Part model, mm, in its own coordinate system. A direction names the side the tool comes from. Give positions to 0.01 mm unless a question says otherwise; leave off trailing zeros. Order: outer loops, then holes, each group sorted by start corner. A loop starts at its lowest first (then second) coordinate and runs counter-clockwise, first axis right, second up. Notation, with made-up numbers: (73.5, -21.5) - (88.5, -21.5) arc R24 cw to (88.5, 10.5) - close; hole circle Ø2 at (31.5, 32). An arc over 180 degrees is marked (long way). Use one line per item in the form item = value. Start each with the question number.
1. Pull direction Z, two halves, no side cores. Call faces 4 (the face through (0, 2, 27.5)), 5 (the face through (10.927, 2, -20)), 6 (the face through (7.25, 2, -11)): +Z half, -Z half, draft (parallel to the pull), parting line (faces both ways), or undercut.
2. Drill centre lines: line 1 (Z direction, x = -7.5, y = 3.6); line 2 (X direction, y = 0.4, z = 5.5). Where is each one in solid material? Low to high.
3. Band-saw the part on A-A, the plane x = -8.25. List the corners of the cut face in (y, z).
4. Band-saw the part on C-C, the plane z = 13. List the corners of the cut face in (x, y).
5. Tool access for faces 1 (the face through (9, 2, -15.5)), 2 (the face through (-9, 2, 14.5)), 3 (the face through (-9, 2, 24.5)): list every direction of +Z, -Z, +X, -X, +Y, -Y with a clear straight run to the whole face (end or side of a thin tool).
6. Pin check, flat tips, straight feed: P1, Ø4, axis at x = -1.5, z = 3, coming from the -Y side; P2, Ø1.9, axis at x = -9.5, y = 1.5, coming from the +Z side; P3, Ø0.9, axis at y = 1, z = 26, coming from the +X side; P4, Ø1.2, axis at y = 2.5, z = -8.5, coming from the -X side. Stop position of each tip, or through.
7. Band-saw the part on B-B, the plane y = 2. List the corners of the cut face in (x, z), plus the area to 3 significant figures.
Autodesk Inventor part; units mm, degrees
ref_plane "YZ Plane" through (0, 0, 0) normal (1, 0, 0) x (0, 1, 0)
ref_plane "XZ Plane" through (0, 0, 0) normal (0, 1, 0) x (-1, 0, 0)
ref_plane "XY Plane" through (0, 0, 0) normal (0, 0, 1) x (1, 0, 0)
sketch "Sketch1" plane through (0, 0, 0) normal (0, 1, 0) x (-1, 0, 0)
  line L0 (-7.25, 27.5) -> (7.25, 27.5)
  line L1 (7.25, 27.5) -> (7.25, -27.5)
  line L2 (7.25, -27.5) -> (-7.25, -27.5)
  line L3 (-7.25, -27.5) -> (-7.25, 27.5)
  line L4 (-7.25, 27.5) -> (7.25, -27.5) construction
  line L5 (7.25, 27.5) -> (-7.25, -27.5) construction
  point P0 (0, 0)
  dimension "d0" = 14.5
  dimension "d1" = 55
extrude "Extrusion1" add sketch "Sketch1" along normal blind 4
sketch "Sketch2" plane through (0, 4, 0) normal (0, 1, 0) x (1, 0, 0)
  line L0 (0, -21.4425) -> (0, 24.9563)
  line L1 (6.9273, -24.5) -> (10.9273, -24.5)
  line L2 (10.9273, -24.5) -> (10.9273, -14.5)
  line L3 (10.9273, -14.5) -> (6.9273, -14.5)
  line L4 (6.9273, -14.5) -> (6.9273, -24.5)
  line L5 (7.25, -27.5) -> (-7.25, -27.5)
  point P0 (0, 0)
  dimension "d10" = 4
  dimension "d11" = 10
  dimension "d12" = 3
extrude "Extrusion2" add sketch "Sketch2" against normal blind 4
pattern_linear "Rectangular Pattern1" count 3 spacing 20 along (0, 0, -1) count 2 spacing 18 along (-1, 0, 0) of "Extrusion2"
properties part number "tussenplaatje"
From the geometry:
q1.face_4 = +Z half
q1.face_5 = draft
q1.face_6 = undercut
q2.line_1 = -25.5 to -15.5, -5.5 to 4.5, 14.5 to 24.5
q2.line_2 = -7.25 to 7.25
q3.outline = (0, -25.5) - (4, -25.5) - (4, -15.5) - (0, -15.5) - close; (0, -5.5) - (4, -5.5) - (4, 4.5) - (0, 4.5) - close; (0, 14.5) - (4, 14.5) - (4, 24.5) - (0, 24.5) - close
q4.outline = (-7.25, 0) - (7.25, 0) - (7.25, 4) - (-7.25, 4) - close
q5.face_1 = +X, +Y, -Y
q5.face_2 = -X, +Y, -Y
q5.face_3 = +Z, -X, +Y, -Y
q6.P1 = 0
q6.P2 = 24.5
q6.P3 = 7.25
q6.P4 = -7.25
q7.outline = (-11.07, -25.5) - (-7.25, -25.5) - (-7.25, -27.5) - (7.25, -27.5) - (7.25, -25.5) - (10.93, -25.5) - (10.93, -15.5) - (7.25, -15.5) - (7.25, -5.5) - (10.93, -5.5) - (10.93, 4.5) - (7.25, 4.5) - (7.25, 14.5) - (10.93, 14.5) - (10.93, 24.5) - (7.25, 24.5) - (7.25, 27.5) - (-7.25, 27.5) - (-7.25, 24.5) - (-11.07, 24.5) - (-11.07, 14.5) - (-7.25, 14.5) - (-7.25, 4.5) - (-11.07, 4.5) - (-11.07, -5.5) - (-7.25, -5.5) - (-7.25, -15.5) - (-11.07, -15.5) - close
q7.area = 1,020 mm²
